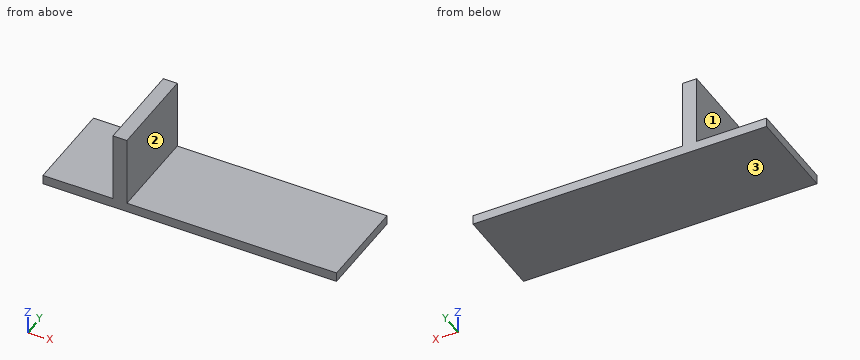
from build123d import *

# Parameters (mm, degrees)
F0_W     = 45
F0_H     = 20
F0_W_2   = 3
F0_W_3   = 15
F1_DEPTH = 2
F2_DEPTH = 15


with BuildPart() as f1:
    # F0 (on Top) → F1 (new body)
    with BuildSketch(Plane.XY):
        with Locations((-21.151677, 21.431452)):
            Rectangle(F0_W, F0_H)
        with Locations((-45.151677, 21.431452)):
            Rectangle(F0_W_2, F0_H)
        with Locations((-54.151677, 21.431452)):
            Rectangle(F0_W_3, F0_H)
    extrude(amount=-F1_DEPTH)

    # F0 (on Top) → F2 (join)
    with BuildSketch(Plane.XY):
        with Locations((-45.151677, 21.431452)):
            Rectangle(F0_W_2, F0_H)
    extrude(amount=F2_DEPTH)


solid = f1.part
Geometry check sheet. Reference: the model listing, model coordinates, mm. Face numbers are marked on the shaded views. A direction names the side the tool comes from. Give positions to 0.01 mm unless a question says otherwise; leave off trailing zeros. Order: outer loops, then holes, each group sorted by start corner. A loop starts at its lowest first (then second) coordinate and runs counter-clockwise, first axis right, second up.
1) Tool access check on the marked faces 1, 2 and 3. Record the directions out of +Z, -Z, +X, -X, +Y, -Y that give a thin tool (end or side, any length) a straight path to the whole face; none if there is none.
Results are:
face 1: +Z, -X, +Y, -Y
face 2: +Z, +X, +Y, -Y
face 3: -Z, +X, -X, +Y, -Y
2) Cross-section at A-A (y = 28). Record the boundary of the cut face in (x, z), then the cut area to 3 significant figures.
Results are:
outline: (-61.65, -2) - (1.35, -2) - (1.35, 0) - (-43.65, 0) - (-43.65, 15) - (-46.65, 15) - (-46.65, 0) - (-61.65, 0) - close
area: 171 mm2
3) Material ranges on probe 1 along X at (y, z) = (28.75, 0.5); probe 2 along Z at (x, y) = (-50, 19.75), recorded low to high.
Results are:
probe 1: x = -46.65 to -43.65
probe 2: z = -2 to 0
4) Cross-section at C-C (x = -20.5). Record the boundary of the cut face in (y, z).
Results are:
outline: (11.43, -2) - (31.43, -2) - (31.43, 0) - (11.43, 0) - close
5) Cross-section at B-B (z = 13.5). Record the boundary of the cut face in (x, y), then the cut area to 3 significant figures.
Results are:
outline: (-46.65, 11.43) - (-43.65, 11.43) - (-43.65, 31.43) - (-46.65, 31.43) - close
area: 60.0 mm2
6) Gauge pin test, flat ends, axial feed: pin 1 (4 mm diameter, centred on x = -43.5, z = 7, fed in from +Y); pin 2 (6 mm diameter, centred on x = -29, y = 19.5, fed in from +Z); pin 3 (5 mm diameter, centred on y = 24.5, z = 7, fed in from +X); pin 4 (10 mm diameter, centred on y = 21.5, z = 7, fed in from -X). Record the tip position at first contact, or that the pin passes through.
Results are:
pin 1: stops at y = 31.43
pin 2: stops at z = 0
pin 3: stops at x = -43.65
pin 4: stops at x = -46.65
